Can you work these out from the model? Positions are in its coordinate system, mm. A direction names the side the tool comes from. Give positions to 0.01 mm unless a question says otherwise; leave off trailing zeros. Order: outer loops, then holes, each group sorted by start corner. A loop starts at its lowest first (then second) coordinate and runs counter-clockwise, first axis right, second up.
```python
from build123d import *

# Parameters (mm, degrees)
SKETCH_R        = 1.75
SKETCH_W        = 15.3
SKETCH_H        = 18
PAD_DEPTH       = 6
SKETCH001_W     = 17
SKETCH001_H     = 19.5
POCKET_DEPTH    = 3
SKETCH002_W     = 0.6
SKETCH002_H     = 4
PAD001_DEPTH    = 1.4
CHAMFER_SIZE    = 0.59
CHAMFER001_SIZE = 1.2


with BuildPart() as part:
    # Sketch → Pad (new body)
    with BuildSketch(Plane.XY):
        with BuildLine():
            Line((-10, 11.25), (10, 11.25))
            Line((10, 11.25), (10, 3.5))
            Line((12.5, 3.5), (10, 3.5))
            ThreePointArc((12.5, -3.5), (16, 0), (12.5, 3.5))
            Line((10, -3.5), (12.5, -3.5))
            Line((10, -3.5), (10, -11.25))
            Line((10, -11.25), (-10, -11.25))
            Line((-10, -11.25), (-10, -3.5))
            Line((-12.5, -3.5), (-10, -3.5))
            ThreePointArc((-12.5, 3.5), (-16, 0), (-12.5, -3.5))
            Line((-10, 3.5), (-12.5, 3.5))
            Line((-10, 3.5), (-10, 11.25))
        make_face()
        with Locations((-12.5, 0)):
            Circle(SKETCH_R, mode=Mode.SUBTRACT)
        with Locations((12.5, 0)):
            Circle(SKETCH_R, mode=Mode.SUBTRACT)
        Rectangle(SKETCH_W, SKETCH_H, mode=Mode.SUBTRACT)
    extrude(amount=PAD_DEPTH)

    # Sketch001 (on Face20 of Pad) → Pocket (cut)
    with BuildSketch(Plane.XY.offset(6)):
        Rectangle(SKETCH001_W, SKETCH001_H)
    extrude(amount=-POCKET_DEPTH, mode=Mode.SUBTRACT)

    # Sketch002 (on Face5 of Pocket) → Pad001 (join)
    with BuildSketch(Plane.XY.offset(6)):
        with Locations((-8.2, 0)):
            Rectangle(SKETCH002_W, SKETCH002_H)
        with Locations((8.2, 0)):
            Rectangle(SKETCH002_W, SKETCH002_H)
    extrude(amount=-PAD001_DEPTH)

    # Chamfer
    chamfer_edges = [part.edges().sort_by_distance(p)[0] for p in [
        (7.9, 0, 6),
        (7.9, 0, 4.6),
        (-7.9, 0, 6),
        (-7.9, 0, 4.6),
    ]]
    chamfer(chamfer_edges, length=CHAMFER_SIZE)

    # Chamfer001
    chamfer001_edges = [part.edges().sort_by_distance(p)[0] for p in [
        (10, -11.25, 3),
    ]]
    chamfer(chamfer001_edges, length=CHAMFER001_SIZE)


solid = part.part
```
1) Suppose I cut it at A-A (y = 6). Please give me the cut outline in (x, z).
2) Which directions (+Z, -Z, +X, -X, +Y, -Y) give clear straight access to the entire face, cutting with the end or side of a thin tool? Please do faces 4 (the face through (-10, -7, 3)), 5 (the face through (0, 9, 1)), 6 (the face through (11, -3.5, 3)), 7 (the face through (10, 7, 3)).
3) If I drill on line 1 (Y direction, x = 0, z = 4.15); line 2 (Y direction, x = 12.5, z = 4.7); line 3 (X direction, y = -8, z = 3.65), over which ranges is the centre line in solid material (lowest first)?
4) I'm going to push flat-ended pins straight in: pin 1 Ø1.5 at (y, z) = (-5, 3.5) entering from +X; pin 2 Ø3.5 at (y, z) = (-2.5, 1.5) entering from -X; pin 3 Ø1.8 at (y, z) = (-9, 4) entering from -X. Where does each tip first touch, or does it pass through?
5) Suppose I cut it at D-D (y = 0). Give the number of separate pieces and of enclosed holes in the cut face, and give its area (3 significant figures).
6) Suppose I cut it at B-B (x = -4.5). Please give me the cut outline in (y, z), and give its area (3 significant figures).
7) We'd pull the mould along Y, two halves only. Please class faces 1 (the face through (0, -11.25, 3)), 2 (the face through (-11, 3.5, 3)), 3 (the face through (7.65, 0, 1)): +Y half, -Y half, draft (parallel to the pull), parting line (faces both ways), or undercut.
8) Suppose I cut it at C-C (z = 3.65). Please give me the cut outline in (x, y), and give its area (3 significant figures).
Results:
1. outline: (-10, 0) - (-7.65, 0) - (-7.65, 3) - (-8.5, 3) - (-8.5, 6) - (-10, 6) - close; (7.65, 0) - (10, 0) - (10, 6) - (8.5, 6) - (8.5, 3) - (7.65, 3) - close
2. face 4: +Z, -Z, -X, -Y
2. face 5: +Z, -Z
2. face 6: +Z, -Z, +X, -Y
2. face 7: +Z, -Z, +X, +Y
3. line 1: y = -11.25 to -9.75, 9.75 to 11.25
3. line 2: y = -3.5 to -1.75, 1.75 to 3.5
3. line 3: x = -10 to -8.5, 8.5 to 10
4. pin 1: stops at x = 10
4. pin 2: stops at x = -15.92
4. pin 3: stops at x = -10
5. separate pieces: 4
5. enclosed holes: 0
5. area: 54.1 mm2
6. outline: (-11.25, 0) - (-9, 0) - (-9, 3) - (-9.75, 3) - (-9.75, 6) - (-11.25, 6) - close; (9, 0) - (11.25, 0) - (11.25, 6) - (9.75, 6) - (9.75, 3) - (9, 3) - close
6. area: 22.5 mm2
7. face 1: -Y half
7. face 2: +Y half
7. face 3: undercut
8. outline: (-12.5, -3.5) - (-10, -3.5) - (-10, -11.25) - (8.8, -11.25) - (10, -10.05) - (10, -3.5) - (12.5, -3.5) arc R3.5 ccw to (12.5, 3.5) - (10, 3.5) - (10, 11.25) - (-10, 11.25) - (-10, 3.5) - (-12.5, 3.5) arc R3.5 ccw to start; hole circle Ø3.5 at (-12.5, 0); hole (-8.5, -9.75) - (8.5, -9.75) - (8.5, 9.75) - (-8.5, 9.75) - close; hole circle Ø3.5 at (12.5, 0)
8. area: 172 mm2
